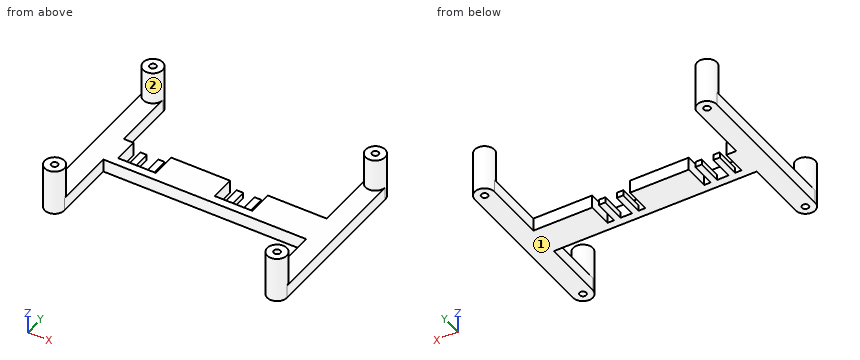
```python
from build123d import *

# Parameters (mm, degrees)
F1_DEPTH = 4
F2_W     = 2
F2_H     = 7.5
F3_DEPTH = 1.7
F5_DEPTH = 10
F6_R     = 1
F7_DEPTH = 25


with BuildPart() as f1:
    # F0 (on Top) → F1 (new body)
    with BuildSketch(Plane.XY):
        with BuildLine():
            Line((6, 0), (68, 0))
            Line((68, 0), (68, -19))
            ThreePointArc((68, -19), (71, -22), (74, -19))
            Line((74, -19), (74, 29))
            ThreePointArc((74, 29), (71, 32), (68, 29))
            Line((68, 29), (68, 10))
            Line((68, 10), (50, 10))
            Line((50, 10), (50, 2.5))
            Line((50, 2.5), (38.5, 2.5))
            Line((38.5, 2.5), (38.5, 10))
            Line((38.5, 10), (20.5, 10))
            Line((20.5, 10), (20.5, 2.5))
            Line((20.5, 2.5), (9, 2.5))
            Line((9, 2.5), (9, 10))
            Line((9, 10), (6, 10))
            Line((6, 10), (6, 29))
            ThreePointArc((6, 29), (3, 32), (0, 29))
            Line((0, 29), (0, -19))
            ThreePointArc((0, -19), (3, -22), (6, -19))
            Line((6, -19), (6, 0))
        make_face()
    extrude(amount=F1_DEPTH)

    # F2 (on Top) → F3 (join)
    with BuildSketch(Plane.XY):
        with Locations((12, 6.25)):
            Rectangle(F2_W, F2_H)
        with Locations((17.5, 6.25)):
            Rectangle(F2_W, F2_H)
        with Locations((41.5, 6.25)):
            Rectangle(F2_W, F2_H)
        with Locations((47, 6.25)):
            Rectangle(F2_W, F2_H)
    extrude(amount=F3_DEPTH)

    # F4 (on face) → F5 (join)
    with BuildSketch(Plane.XY.offset(4)):
        with BuildLine():
            ThreePointArc((0, 29), (3, 26), (6, 29))
            ThreePointArc((6, 29), (3, 32), (0, 29))
        make_face()
        with BuildLine():
            ThreePointArc((6, -19), (3, -16), (0, -19))
            ThreePointArc((0, -19), (3, -22), (6, -19))
        make_face()
        with BuildLine():
            ThreePointArc((74, -19), (71, -16), (68, -19))
            ThreePointArc((68, -19), (71, -22), (74, -19))
        make_face()
        with BuildLine():
            ThreePointArc((68, 29), (71, 26), (74, 29))
            ThreePointArc((74, 29), (71, 32), (68, 29))
        make_face()
    extrude(amount=F5_DEPTH)

    # F6 (on face) → F7 (cut)
    with BuildSketch(Plane(origin=(0, 0, 0), x_dir=(1, 0, 0), z_dir=(0, 0, -1))):
        with Locations((3, 19)):
            Circle(F6_R)
        with Locations((71, 19)):
            Circle(F6_R)
        with Locations((71, -29)):
            Circle(F6_R)
        with Locations((3, -29)):
            Circle(F6_R)
    extrude(amount=-F7_DEPTH, mode=Mode.SUBTRACT)


solid = f1.part
```
The model under review builds one solid part; all positions refer to its coordinate system, in mm. Face numbers are marked on the shaded views. Round coordinates to 2 decimals unless told otherwise and drop trailing zeros. Loops run counter-clockwise (first coordinate to the right, second up) from the corner with the lowest first, then second, coordinate; pieces in that order, holes last. Notation, with made-up numbers: (77.25, 47) - (133.25, 47) arc R22 cw to (133.25, 81) - close; hole circle Ø6 at (-26, 76.5). An arc over 180 degrees is marked (long way). Write each question's results on one line, items separated by ' | '. Start each with the question number.
Q1. Insertion check: P1, Ø1.4, axis at x = 47, z = 1, coming from the +Y side; P2, Ø12, axis at x = 34.5, y = 0.5, coming from the +Z side; P3, Ø3, axis at x = 71, y = 29, coming from the +Z side; P4, Ø2, axis at x = 39.5, z = 4.5, coming from the +Y side. Each pin has a flat end and moves straight along its axis. Give the tip position at first contact, or say it passes through.
Q2. Take a section at D-D on y = 27. Give the boundary of the cut face in (x, z), plus the area to 3 significant figures.
Q3. Take a section at B-B on x = 3. Give the boundary of the cut face in (y, z).
Q4. Take a section at C-C on y = 14. Give the boundary of the cut face in (x, z).
Q5. Take a section at A-A on z = 8. Give the boundary of the cut face in (x, y).
Q6. Wall thickness on line 1 along Y through (x, z) = (3, 3.25); line 2 along X through (y, z) = (-19, 10.5); line 3 along Y through (x, z) = (3, 6.75): over which ranges is each line inside the solid? List them lowest first. Write a range as [from, to].
Q7. Draft analysis for pull direction X (two halves, no side actions). For the marked faces 1 and 2, state which applies: pulls with the +X half, pulls with the -X half, needs draft (parallel to the pull), parting line crosses it, or undercut.
Data:
1) P1: stops at y = 10 | P2: stops at z = 4 | P3: stops at z = 14 | P4: stops at y = 2.5
2) outline: (0, 0) - (6, 0) - (6, 4) - (5.24, 4) - (5.24, 14) - (0.76, 14) - (0.76, 4) - (0, 4) - close; (68, 0) - (74, 0) - (74, 4) - (73.24, 4) - (73.24, 14) - (68.76, 14) - (68.76, 4) - (68, 4) - close | area: 137 mm²
3) outline: (-22, 0) - (-20, 0) - (-20, 14) - (-22, 14) - close; (-18, 0) - (28, 0) - (28, 14) - (26, 14) - (26, 4) - (-16, 4) - (-16, 14) - (-18, 14) - close; (30, 0) - (32, 0) - (32, 14) - (30, 14) - close
4) outline: (0, 0) - (6, 0) - (6, 4) - (0, 4) - close; (68, 0) - (74, 0) - (74, 4) - (68, 4) - close
5) outline: circle Ø6 at (3, -19); circle Ø6 at (3, 29); circle Ø6 at (71, -19); circle Ø6 at (71, 29); hole circle Ø2 at (3, -19); hole circle Ø2 at (3, 29); hole circle Ø2 at (71, -19); hole circle Ø2 at (71, 29)
6) line 1: y = [-22, -20], [-18, 28], [30, 32] | line 2: x = [0, 2], [4, 6], [68, 70], [72, 74] | line 3: y = [-22, -20], [-18, -16], [26, 28], [30, 32]
7) face 1: needs draft | face 2: undercut
